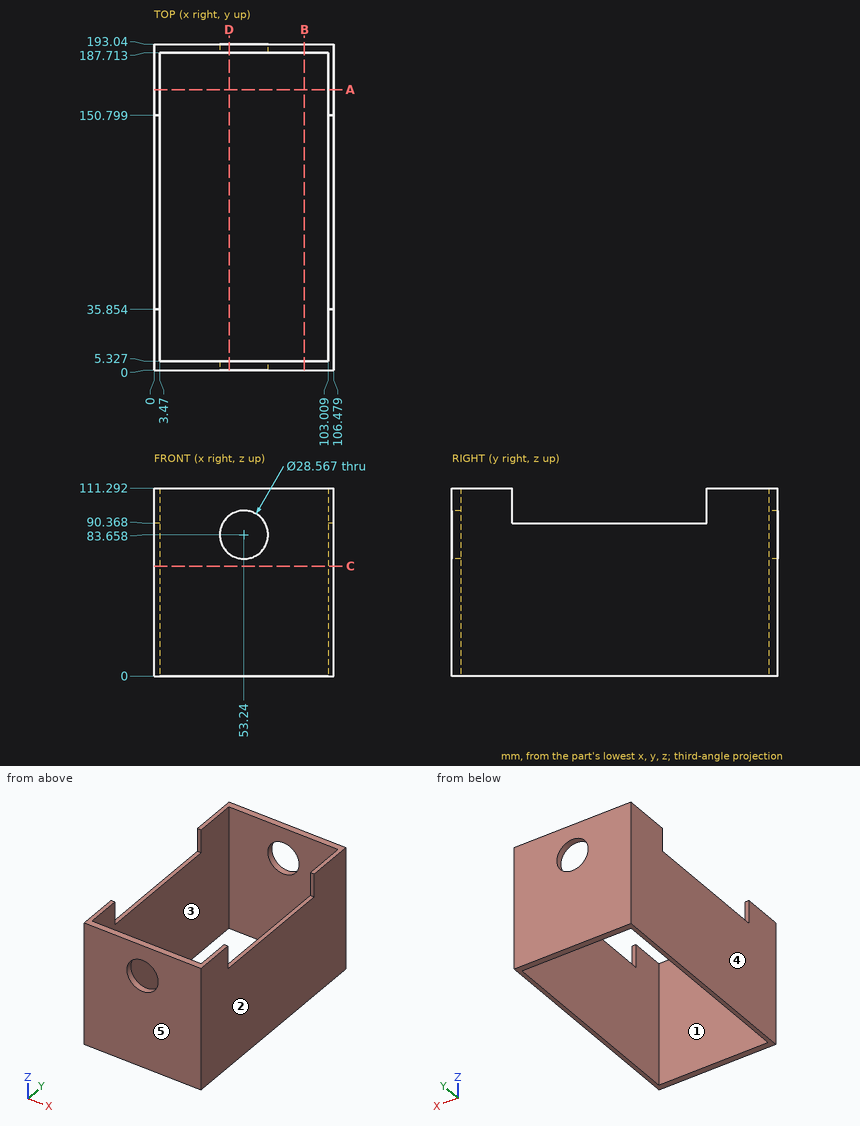
Study the drawing (mm; zero at the part's minimum x, y, z) and answer. A direction names the side the tool comes from. Round coordinates to 2 decimals unless told otherwise and drop trailing zeros. Loops run counter-clockwise (first coordinate to the right, second up) from the corner with the lowest first, then second, coordinate; pieces in that order, holes last.
Q1. Which of the six approach directions +Z, -Z, +X, -X, +Y, -Y give full straight-line access (tool end or side, diameter ignored) to the marked faces 1 and 2?
Q2. Section D-D, the plane x = 44.5 is taken. Determine the outline of the cut face in (y, z).
Q3. Section C-C, the plane z = 65 is taken. Determine the outline of the cut face in (x, y), then the cut area to 3 significant figures.
Q4. Section A-A, the plane y = 166 is taken. Determine the outline of the cut face in (x, z).
Q5. Given pin 1 Ø4 at (x, y) = (2, 92) entering from +Z, flat-ended and moving along its own axis, determine where the tip first touches the part or whether it passes through.
Q6. Find the intervals of material crossed by line 1 (X direction, y = 41, z = 5); line 2 (Y direction, x = 31, z = 52), in increasing order.
Q7. For a pull along Y with two mould halves and no side action, classify the marked faces 3, 4 and 5 as released by +Y, released by -Y, zero draft, split by the parting line, or undercut.
Q8. Section B-B, the plane x = 89 is taken. Determine the outline of the cut face in (y, z), then the cut area to 3 significant figures.
Completed:
1. face 1: +Z, -Z
1. face 2: +Z, -Z, +X, +Y, -Y
2. outline: (0, 0) - (5.33, 0) - (5.33, 72.36) - (0, 72.36) - close; (0, 94.96) - (5.33, 94.96) - (5.33, 111.29) - (0, 111.29) - close; (187.71, 0) - (193.04, 0) - (193.04, 72.36) - (187.71, 72.36) - close; (187.71, 94.96) - (193.04, 94.96) - (193.04, 111.29) - (187.71, 111.29) - close
3. outline: (0, 0) - (106.48, 0) - (106.48, 193.04) - (0, 193.04) - close; hole (3.47, 5.33) - (103.01, 5.33) - (103.01, 187.71) - (3.47, 187.71) - close
3. area: 2,400 mm2
4. outline: (0, 0) - (3.47, 0) - (3.47, 111.29) - (0, 111.29) - close; (103.01, 0) - (106.48, 0) - (106.48, 111.29) - (103.01, 111.29) - close
5. pin 1: stops at z = 90.37
6. line 1: x = 0 to 3.47, 103.01 to 106.48
6. line 2: y = 0 to 5.33, 187.71 to 193.04
7. face 3: undercut
7. face 4: zero draft
7. face 5: released by -Y
8. outline: (0, 0) - (5.33, 0) - (5.33, 111.29) - (0, 111.29) - close; (187.71, 0) - (193.04, 0) - (193.04, 111.29) - (187.71, 111.29) - close
8. area: 1,190 mm2
